from build123d import *

# Parameters (mm, degrees)
CYLINDER_R     = 2.5
CYLINDER_DEPTH = 50


with BuildPart() as cone:
    # Cone → Cone (revolve)
    with BuildSketch(Plane(origin=(0, 0, -3), x_dir=(1, 0, 0), z_dir=(0, -1, 0))):
        Polygon((0, 0), (4.5, 0), (2.5, 3), (0, 3), align=None)
    revolve(axis=Axis((0, 0, -3), (0, 0, 1)))


with BuildPart() as obj1:
    # Cylinder → Cylinder (new body)
    with BuildSketch(Plane.XY):
        Circle(CYLINDER_R)
    extrude(amount=CYLINDER_DEPTH)

    # Fusion: union Cone
    add(cone.part)


solid = obj1.part
The model under review builds one solid part; all positions refer to its coordinate system, in mm. A direction names the side the tool comes from. Coordinates: 2 decimals unless noted, no trailing zeros. Loops run counter-clockwise (first coordinate to the right, second up) from the corner with the lowest first, then second, coordinate; pieces in that order, holes last. Notation, with made-up numbers: M 69,-8 L 95,-8 A8 ccw 95,5 Z; hole C 9,-25.75 d11. An arc over 180 degrees is marked long. Put each result on its own line as item: value. Start each with the question number.
Q1. Wall thickness on line 1 (Y direction, x = 0, z = 2); line 2 (X direction, y = 2.25, z = 47.5); line 3 (X direction, y = -1, z = 37): over which ranges is each line inside the solid? List them lowest first.
Q2. Add section A-A (y = 0). Write out the cut boundary in (x, z).
Q3. Clearance check with flat-ended pins moving along their axes: pin 1 (2 mm diameter, centred on y = 3, z = 4, fed in from +X); pin 2 (2 mm diameter, centred on y = -2.5, z = 24.5, fed in from -X); pin 3 (3 mm diameter, centred on y = -2.5, z = 3, fed in from +X). State where each tip first meets the part, or that it passes through.
Q4. Add section C-C (z = 23.5). Write out the cut boundary in (x, y).
Q5. For faces 1 (the cylindrical face through (-0.54, -2.44, 24.65)), 2 (the flat face through (0, 0, 50)), list the 3-axis set-ups (+Z, -Z, +X, -X, +Y, -Y) from which the entire face can be reached by the end or side of a thin tool; tool diameter is ignored.
Answers:
1. line 1: y = -2.5 to 2.5
1. line 2: x = -1.09 to 1.09
1. line 3: x = -2.29 to 2.29
2. outline: M -4.5,-3 L 4.5,-3 L 2.5,0 L 2.5,50 L -2.5,50 L -2.5,0 Z
3. pin 1: stops at x = 1.5
3. pin 2: stops at x = -2
3. pin 3: stops at x = 2.29
4. outline: C 0,0 d5
5. face 1: +Z
5. face 2: +Z, +X, -X, +Y, -Y
